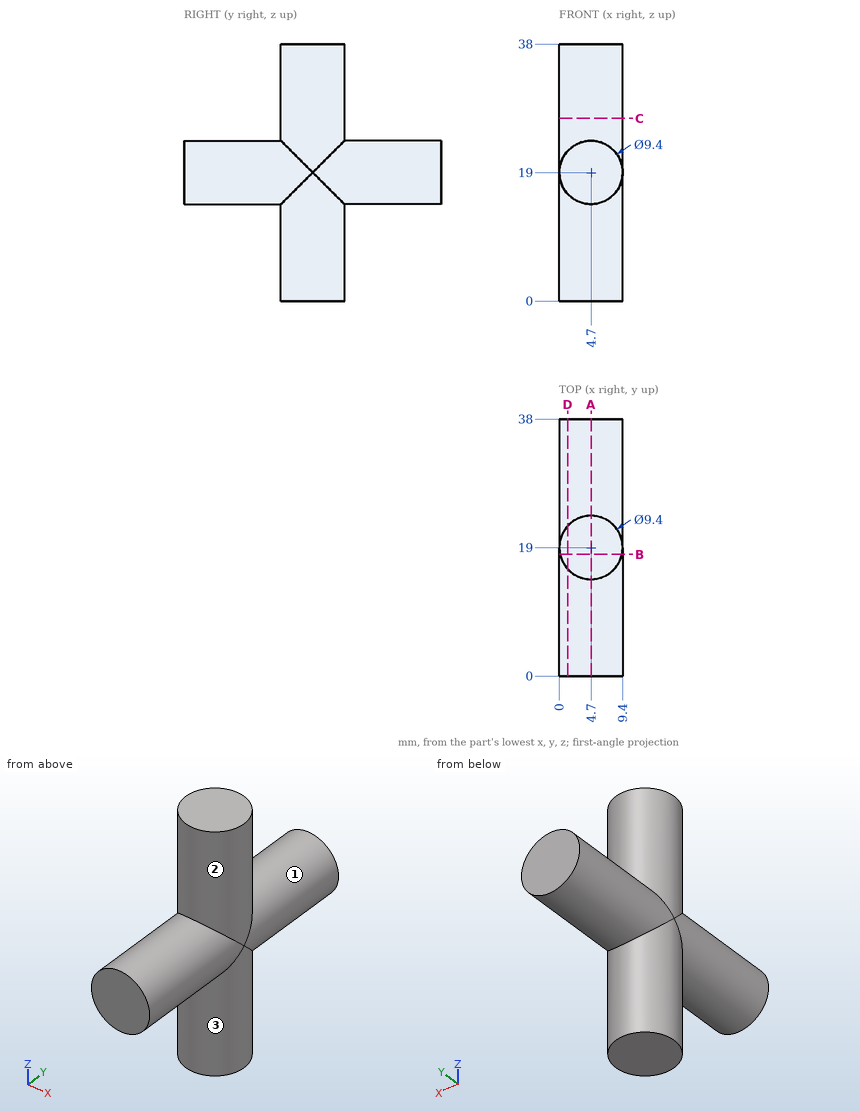
Geometry check sheet. Reference: drawing and pictorial views, mm from the part's lowest x, y, z. A direction names the side the tool comes from. Round coordinates to 2 decimals unless told otherwise and drop trailing zeros. Loops run counter-clockwise (first coordinate to the right, second up) from the corner with the lowest first, then second, coordinate; pieces in that order, holes last. Notation, with made-up numbers: (47, 60) - (63, 60) arc R25 cw to (63, 99) - close; hole circle Ø5 at (57, 74.5). An arc over 180 degrees is marked (long way). Write item = value, one per line. Start each with the question number.
Q1. Thickness scan on L1, parallel to Z at x = 4.5, y = 32; L2, parallel to X at y = 20, z = 5; L3, parallel to X at y = 21, z = 32.5. Record the ranges inside material, lowest first.
Q2. Section check C-C (z = 27). Record the boundary of the cut face in (x, y), plus the area to 3 significant figures.
Q3. Section check A-A (x = 4.7). Record the boundary of the cut face in (y, z).
Q4. Section check D-D (x = 1.25). Record the boundary of the cut face in (y, z).
Q5. Depth check by flat-ended pin: P1, Ø1.5, axis at y = 12.5, z = 15.5, coming from the -X side; P2, Ø1.5, axis at x = 7, y = 10.5, coming from the -Z side; P3, Ø5, axis at y = 30, z = 27.5, coming from the -X side. Enter the tip coordinate at first touch or a pass-through.
Q6. Access from +Z, -Z, +X, -X, +Y, -Y to the whole of each face (thin tool, end or side, straight path). Record for the marked faces 1, 2 and 3.
Q7. Section check B-B (y = 18). Record the boundary of the cut face in (x, z), plus the area to 3 significant figures.
Derived:
q1.L1 = 14.3 to 23.7
q1.L2 = 0.11 to 9.29
q1.L3 = 0.45 to 8.95
q2.outline = circle Ø9.4 at (4.7, 19)
q2.area = 69.4 mm^2
q3.outline = (0, 14.3) - (14.3, 14.3) - (14.3, 0) - (23.7, 0) - (23.7, 14.3) - (38, 14.3) - (38, 23.7) - (23.7, 23.7) - (23.7, 38) - (14.3, 38) - (14.3, 23.7) - (0, 23.7) - close
q4.outline = (0, 15.81) - (15.81, 15.81) - (15.81, 0) - (22.19, 0) - (22.19, 15.81) - (38, 15.81) - (38, 22.19) - (22.19, 22.19) - (22.19, 38) - (15.81, 38) - (15.81, 22.19) - (0, 22.19) - close
q5.P1 = 0.89
q5.P2 = 14.56
q5.P3 = through
q6.face_1 = +Y
q6.face_2 = +Z
q6.face_3 = -Z
q7.outline = (0.11, 0) - (9.29, 0) - (9.29, 18) arc R4.7 ccw to (9.29, 20) - (9.29, 38) - (0.11, 38) - (0.11, 20) arc R4.7 ccw to (0.11, 18) - close
q7.area = 349 mm^2
